Could you check a few things on this model? Use its own coordinates, in mm. Face numbers are marked on the shaded views. Coordinates: 2 decimals unless noted, no trailing zeros. Loops run counter-clockwise (first coordinate to the right, second up) from the corner with the lowest first, then second, coordinate; pieces in that order, holes last. Notation, with made-up numbers: M -39.5,75.25 L -30.5,75.25 A24 ccw -30.5,110.25 Z; hole C -25,46.25 d6. An arc over 180 degrees is marked long. Write each question's results on one line, items separated by ' | '.
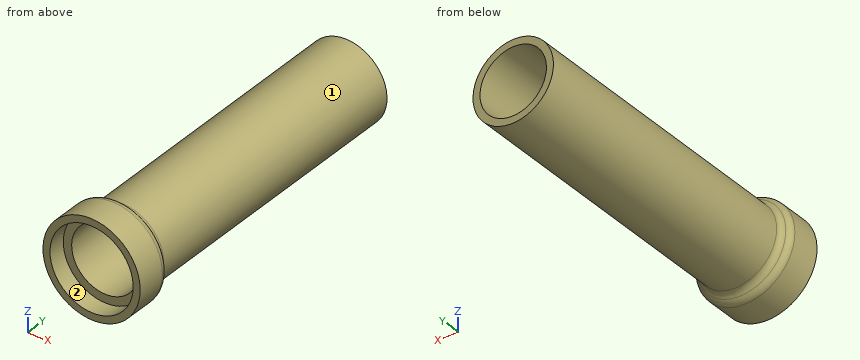
```python
from build123d import *

# Parameters (mm, degrees)
SKETCH1_R           = 17.653
SKETCH1_R_2         = 15.113
BOSS_EXTRUDE1_DEPTH = 6.35
SKETCH2_R           = 17.653
SKETCH2_R_2         = 12.065
BOSS_EXTRUDE2_DEPTH = 6.35
SKETCH3_R           = 14.605
SKETCH3_R_2         = 12.065
BOSS_EXTRUDE3_DEPTH = 109.22
FILLET1_R           = 2.54
FILLET2_R           = 2.54


with BuildPart() as part:
    # Sketch1 → Boss-Extrude1 (new body)
    with BuildSketch(Plane(origin=(0, 0, 0), x_dir=(1, 0, 0), z_dir=(0, 1, 0))):
        with Locations(Location((0, 0, 0), (0, 0, 270))):
            Circle(SKETCH1_R)
        with Locations(Location((0, 0, 0), (0, 0, 270))):
            Circle(SKETCH1_R_2, mode=Mode.SUBTRACT)
    extrude(amount=BOSS_EXTRUDE1_DEPTH)

    # Sketch2 → Boss-Extrude2 (add)
    with BuildSketch(Plane(origin=(0, 6.35, 0), x_dir=(1, 0, 0), z_dir=(0, 1, 0))):
        with Locations(Location((0, 0, 0), (0, 0, 270))):
            Circle(SKETCH2_R)
        with Locations(Location((0, 0, 0), (0, 0, 270))):
            Circle(SKETCH2_R_2, mode=Mode.SUBTRACT)
    extrude(amount=BOSS_EXTRUDE2_DEPTH)

    # Sketch3 → Boss-Extrude3 (add)
    with BuildSketch(Plane(origin=(0, 12.7, 0), x_dir=(1, 0, 0), z_dir=(0, 1, 0))):
        with Locations(Location((0, 0, 0), (0, 0, 270))):
            Circle(SKETCH3_R)
        with Locations(Location((0, 0, 0), (0, 0, 270))):
            Circle(SKETCH3_R_2, mode=Mode.SUBTRACT)
    extrude(amount=BOSS_EXTRUDE3_DEPTH)

    # Fillet1
    fillet1_edges = [part.edges().sort_by_distance(p)[0] for p in [
        (0, 12.7, -14.605),
    ]]
    fillet(fillet1_edges, radius=FILLET1_R)

    # Fillet2
    fillet2_edges = [part.edges().sort_by_distance(p)[0] for p in [
        (0, 12.7, -17.653),
    ]]
    fillet(fillet2_edges, radius=FILLET2_R)


solid = part.part
```
(1) Will these pins go through, and if not, where does the flat tip stop? P1, Ø8, axis at x = -1.5, y = 104, coming from the +Z side (3 decimals); P2, Ø2, axis at x = -2.5, y = 57.5, coming from the -Z side; P3, Ø8, axis at x = -0.5, z = -10.5, coming from the +Y side; P4, Ø6, axis at x = -11.5, y = 47.5, coming from the -Z side.
Reported:
P1: stops at z = 14.605 | P2: stops at z = -14.53 | P3: stops at y = 121.92 | P4: stops at z = -11.88
(2) If we mould it in two halves opening along Z, with no side actions, what happens to the marked faces 1 and 2? For each: released by +Z, released by -Z, zero draft, split by the parting line, or undercut.
Reported:
face 1: split by the parting line | face 2: undercut
(3) Imagine slicing it at A-A, the plane y = 45. List the corners of the cut face in (x, z) for me (3 decimals).
Reported:
outline: C 0,0 d29.21; hole C 0,0 d24.13
(4) Please list where these lines run through material, in increasing order: probe 1 along X at (y, z) = (44.5, 0) (3 decimals); probe 2 along X at (y, z) = (4.25, 0); probe 3 along Z at (x, y) = (5.5, 79). Write a range as from..to.
Reported:
probe 1: x = -14.605..-12.065, 12.065..14.605 | probe 2: x = -17.65..-15.11, 15.11..17.65 | probe 3: z = -13.53..-10.74, 10.74..13.53
